Design review of the part built by this model. Coordinates are the model's own, in mm. Face numbers are marked on the shaded views. Give positions to 0.01 mm unless a question says otherwise; leave off trailing zeros. Write each loop counter-clockwise with the first axis right and the second up, starting at its lowest first coordinate (ties: lowest second). Pieces come first, ordered by that corner, then holes. Notation, with made-up numbers: M -30.75,39 L -18.75,39 A15 cw -18.75,66 Z; hole C 18,38.25 d2. An arc over 180 degrees is marked long. Write each question's results on one line, items separated by ' | '. Start each with the question number.
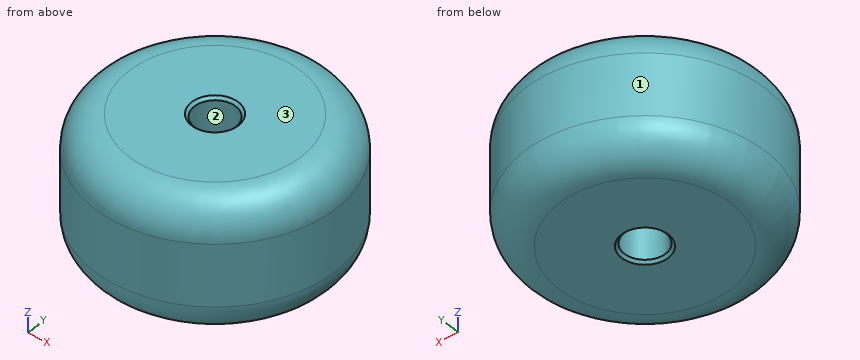
from build123d import *

# Parameters (mm, degrees)
SKETCH_1_R      = 17.5
SKETCH_1_R_2    = 3
EXTRUDE_1_DEPTH = 9.5
FILLET_1_R      = 5
CHAMFER_1_SIZE  = 0.4


with BuildPart() as part:
    # 草图1 → 凸台-拉伸1 (new, symmetric)
    with BuildSketch(Plane.XY):
        Circle(SKETCH_1_R)
        Circle(SKETCH_1_R_2, mode=Mode.SUBTRACT)
    extrude(amount=EXTRUDE_1_DEPTH, both=True)

    # 圆角1
    fillet_1_edges = [part.edges().sort_by_distance(p)[0] for p in [
        (-17.5, 0, -9.5),
        (-17.5, 0, 9.5),
    ]]
    fillet(fillet_1_edges, radius=FILLET_1_R)

    # 倒角1
    chamfer_1_edges = [part.edges().sort_by_distance(p)[0] for p in [
        (-3, 0, -9.5),
        (-3, 0, 9.5),
    ]]
    chamfer(chamfer_1_edges, length=CHAMFER_1_SIZE)


solid = part.part
Q1. Wall thickness on line 1 along Y through (x, z) = (0, -4); line 2 along X through (y, z) = (1.5, 5); line 3 along Z through (x, y) = (-13.5, -6): over which ranges is each line inside the solid? List them lowest first. Write a range as from..to.
Q2. We need section A-A on x = 0. Write out the cut boundary in (y, z), and give its area (3 significant figures).
Q3. We need section C-C on z = 3. Write out the cut boundary in (x, y).
Q4. We need section D-D on z = -7.25. Write out the cut boundary in (x, y), and give its area (3 significant figures).
Q5. For pin 1 Ø3 at (x, y) = (10.5, 11) entering from -Z; pin 2 Ø4 at (y, z) = (-8, 2.5) entering from +X; pin 3 Ø5 at (x, y) = (0, 0) entering from +Z; pin 4 Ø4 at (y, z) = (-9.5, 4.5) entering from -X, all flat-tipped, find the tip position at first contact; note any pin that passes through.
Q6. The part is to be moulded in two halves that separate along X. For the marked faces 1, 2 and 3, say which applies: pulls with the +X half, pulls with the -X half, needs draft (parallel to the pull), parting line crosses it, or undercut.
Answer sheet:
1) line 1: -17.5..-3, 3..17.5 | line 2: -17.41..-2.6, 2.6..17.41 | line 3: -8.95..8.95
2) outline: M -17.5,-4.5 A5 ccw -12.5,-9.5 L -3.4,-9.5 L -3,-9.1 L -3,9.1 L -3.4,9.5 L -12.5,9.5 A5 ccw -17.5,4.5 Z; M 3,-9.1 L 3.4,-9.5 L 12.5,-9.5 A5 ccw 17.5,-4.5 L 17.5,4.5 A5 ccw 12.5,9.5 L 3.4,9.5 L 3,9.1 Z | area: 529 mm^2
3) outline: C 0,0 d35; hole C 0,0 d6
4) outline: C 0,0 d33.35; hole C 0,0 d6 | area: 845 mm^2
5) pin 1: z = -9.35 | pin 2: x = 16.44 | pin 3: through | pin 4: x = -15.81
6) face 1: parting line crosses it | face 2: undercut | face 3: needs draft
